from build123d import *

# Parameters (mm, degrees)
F0_R      = 10
F1_DEPTH  = 5
F2_SIZE   = 1.5
F3_R      = 1.5
F4_DEPTH  = 2
F6_DEPTH  = 12.5
F7_R      = 0.75
F10_DEPTH = 1
F11_DEPTH = 1
F12_R     = 0.5


with BuildPart() as f1:
    # F0 (on Top) → F1 (new body)
    with BuildSketch(Plane.XY):
        Circle(F0_R)
    extrude(amount=F1_DEPTH)

    # F2
    f2_edges = [f1.edges().sort_by_distance(p)[0] for p in [
        (-10, 0, 5),
    ]]
    chamfer(f2_edges, length=F2_SIZE)

    # F3 (on face) → F4 (join)
    with BuildSketch(Plane.XY.offset(5)):
        with Locations((-5, 0)):
            Circle(F3_R)
        with Locations((5, 0)):
            Circle(F3_R)
    extrude(amount=F4_DEPTH)

    # F5 (on face) → F6 (join)
    with BuildSketch(Plane.XY.offset(7)):
        Polygon((-7.5213718601, 2.4349466817), (-7.4997186786, -0.0649595445), (-7.4780654971, -2.5648657707), (7.5213718601, -2.4349466817), (7.4780654971, 2.5648657707), align=None)
        with BuildLine():
            ThreePointArc((-3.5, 0), (-3.5000766094, -0.015159897), (-3.50030643, -0.0303182454))
            ThreePointArc((-3.50030643, -0.0303182454), (-4.9870080911, -1.4999437357), (-6.4989433936, -0.0562912318))
            ThreePointArc((-6.4989433936, -0.0562912318), (-5.0281505737, 1.4997358251), (-3.5, 0))
        make_face(mode=Mode.SUBTRACT)
        with BuildLine():
            Line((-6.4989433936, -0.0562912318), (-3.50030643, -0.0303182454))
            ThreePointArc((-3.50030643, -0.0303182454), (-3.5000766094, -0.015159897), (-3.5, 0))
            ThreePointArc((-3.5, 0), (-5.0281505737, 1.4997358251), (-6.4989433936, -0.0562912318))
        make_face()
        with BuildLine():
            ThreePointArc((-6.4989433936, -0.0562912318), (-4.9870080911, -1.4999437357), (-3.50030643, -0.0303182454))
            Line((-3.50030643, -0.0303182454), (-6.4989433936, -0.0562912318))
        make_face()
    extrude(amount=F6_DEPTH)

    # F7
    f7_edges = [f1.edges().sort_by_distance(p)[0] for p in [
        (0.021653, -2.499906, 7),
        (7.521372, -2.434947, 13.25),
        (-7.478065, -2.564866, 13.25),
        (-7.521372, 2.434947, 13.25),
        (-7.499719, -0.06496, 7),
        (-7.499719, -0.06496, 19.5),
        (-0.021653, 2.499906, 19.5),
        (0.021653, -2.499906, 19.5),
        (7.499719, 0.06496, 19.5),
        (7.478065, 2.564866, 13.25),
        (7.499719, 0.06496, 7),
        (-0.021653, 2.499906, 7),
    ]]
    fillet(f7_edges, radius=F7_R)

    # F9 (on offset) → F10 (join)
    with BuildSketch(Plane(origin=(0, 0, 0), x_dir=(-0.9999624905, -0.0086612726, 0), z_dir=(-0.0086612726, 0.9999624905, 0))):
        with BuildLine():
            ThreePointArc((-1.5, 19.5), (0, 21), (1.5, 19.5))
            Line((1.5, 19.5), (2.5, 19.5))
            ThreePointArc((2.5, 19.5), (0, 22), (-2.5, 19.5))
            Line((-2.5, 19.5), (-1.5, 19.5))
        make_face()
    extrude(amount=F10_DEPTH)

    # F11 (add): a face of the model
    f11_faces = [f1.faces().sort_by_distance(p)[0] for p in [
        (0, 0, 21.0559016994),
    ]]
    extrude(f11_faces, amount=F11_DEPTH)

    # F12
    f12_edges = [f1.edges().sort_by_distance(p)[0] for p in [
        (-0.008661, 0.999962, 22),
        (0.008661, -0.999962, 22),
    ]]
    fillet(f12_edges, radius=F12_R)


solid = f1.part
Here's how the part is built. I have some questions about the finished solid (model axes, mm). A direction names the side the tool comes from. Give positions to 0.01 mm unless a question says otherwise; leave off trailing zeros. Order: outer loops, then holes, each group sorted by start corner. A loop starts at its lowest first (then second) coordinate and runs counter-clockwise, first axis right, second up. Notation, with made-up numbers: M 87,-39.5 L 121,-39.5 A30 ccw 121,-0.5 Z; hole C -36.5,-10.5 d5. An arc over 180 degrees is marked long. Answer as a JSON object with one key per item and string values. Group by question number.
1) Suppose I cut it at A-A, the plane z = 13.75. Write out the boundary of the cut face in (x, y), plus the area to 3 significant figures.
2) We'd pull the mould along X, two halves only. Please class faces 6 (the flat face through (0, 0, 7)), 7 (the cylindrical face through (-2.17, -9.76, 1.73)), 8 (the flat face through (0, 0, 0)): pulls with the +X half, pulls with the -X half, needs draft (parallel to the pull), parting line crosses it, or undercut.
3) On a 3-axis mill with a long thin cutter (end or side, diameter ignored), from which of +Z, -Z, +X, -X, +Y, -Y can I reach the whole of each face in a straight line? I mean faces 1 (the cylindrical face through (0.11, -2.29, 7.23)), 2 (the cylindrical face through (-0.11, 2.29, 7.23)), 3 (the cylindrical face through (-0.11, 2.29, 19.27)), 4 (the cylindrical face through (-6.2, -0.9, 6)), 5 (the cylindrical face through (0.11, -2.29, 19.27)). Say none if no direction works.
4) Suppose I cut it at B-B, the plane x = -0.5. Count the separate pieces of the cut face and the enclosed holes in it, plus the area to 3 significant figures.
5) I'm going to push flat-ended pins straight in: pin 1 Ø1.5 at (y, z) = (-4.5, 9) entering from -X; pin 2 Ø10 at (x, z) = (8, 14.5) entering from -Y; pin 3 Ø1 at (y, z) = (-0.5, 13.5) entering from +X; pin 4 Ø2 at (x, y) = (-7.5, -7.5) entering from +Z. Where does each tip first touch, or does it pass through?
6) Please list where these lines run through material, in increasing order: L1, parallel to Y at x = -0.25, z = 3; L2, parallel to Z at x = -3.25, y = 1.5; L3, parallel to Y at x = -6.5, z = 8.5. Write a range as [from, to].
Results found:
{
 "1": {"outline": "M -7.51,1.68 L -7.48,-1.81 A0.75 ccw -6.73,-2.56 L 6.77,-2.44 A0.75 ccw 7.51,-1.68 L 7.48,1.81 A0.75 ccw 6.73,2.56 L -6.77,2.44 A0.75 ccw Z", "area": "74.5 mm²"},
 "2": {"face 6": "undercut", "face 7": "parting line crosses it", "face 8": "needs draft"},
 "3": {"face 1": "+X, -Y", "face 2": "-X, +Y", "face 3": "+Z, -X, +Y", "face 4": "none", "face 5": "+Z, +X, -Y"},
 "4": {"separate pieces": "3", "enclosed holes": "0", "area": "162 mm²"},
 "5": {"pin 1": "through", "pin 2": "y = -2.47", "pin 3": "x = 7.51", "pin 4": "z = 3.89"},
 "6": {"L1": "[-10, 10]", "L2": "[0, 5], [7, 19.5]", "L3": "[-2.56, 2.44]"}
}
